from build123d import *

# Parameters (mm, degrees)
SKETCH1_W           = 41.2
SKETCH1_H           = 42
BOSS_EXTRUDE1_DEPTH = 5
CUT_EXTRUDE1_DEPTH  = 3
CUT_EXTRUDE2_DEPTH  = 2
SKETCH8_W           = 7.25
SKETCH8_H           = 6
BOSS_EXTRUDE4_DEPTH = 8
SKETCH9_W           = 7.25
SKETCH9_H           = 6
BOSS_EXTRUDE5_DEPTH = 8
SKETCH12_R          = 2
CUT_EXTRUDE4_DEPTH  = 6
BOSS_EXTRUDE6_DEPTH = 7.25
FILLET1_R           = 2
FILLET2_R           = 2


with BuildPart() as part:
    # Sketch1 → Boss-Extrude1 (new body)
    with BuildSketch(Plane.XY):
        with Locations((20.6, -21)):
            Rectangle(SKETCH1_W, SKETCH1_H)
    extrude(amount=BOSS_EXTRUDE1_DEPTH)

    # Sketch2 → Cut-Extrude1 (cut)
    with BuildSketch(Plane.XY.offset(5)):
        with BuildLine():
            Line((4, -2), (37.2, -2))
            ThreePointArc((37.2, -2), (38.614213562, -2.585786438), (39.2, -4))
            Line((39.2, -4), (39.2, -38))
            ThreePointArc((39.2, -38), (38.614213562, -39.414213562), (37.2, -40))
            Line((37.2, -40), (4, -40))
            ThreePointArc((4, -40), (2.585786438, -39.414213562), (2, -38))
            Line((2, -38), (2, -4))
            ThreePointArc((2, -4), (2.585786438, -2.585786438), (4, -2))
        make_face()
    extrude(amount=-CUT_EXTRUDE1_DEPTH, mode=Mode.SUBTRACT)

    # Sketch3 → Cut-Extrude2 (cut)
    with BuildSketch(Plane.XY.offset(2)):
        with BuildLine():
            Line((9.25, -7.25), (31.95, -7.25))
            ThreePointArc((31.95, -7.25), (33.364213562, -7.835786438), (33.95, -9.25))
            Line((33.95, -9.25), (33.95, -14.15))
            ThreePointArc((33.95, -14.15), (33.364213562, -15.564213562), (31.95, -16.15))
            Line((31.95, -16.15), (9.25, -16.15))
            ThreePointArc((9.25, -16.15), (7.835786438, -15.564213562), (7.25, -14.15))
            Line((7.25, -14.15), (7.25, -9.25))
            ThreePointArc((7.25, -9.25), (7.835786438, -7.835786438), (9.25, -7.25))
        make_face()
        with BuildLine():
            Line((9.25, -25.85), (31.95, -25.85))
            ThreePointArc((31.95, -25.85), (33.364213562, -26.435786438), (33.95, -27.85))
            Line((33.95, -27.85), (33.95, -32.75))
            ThreePointArc((33.95, -32.75), (33.364213562, -34.164213562), (31.95, -34.75))
            Line((31.95, -34.75), (9.25, -34.75))
            ThreePointArc((9.25, -34.75), (7.835786438, -34.164213562), (7.25, -32.75))
            Line((7.25, -32.75), (7.25, -27.85))
            ThreePointArc((7.25, -27.85), (7.835786438, -26.435786438), (9.25, -25.85))
        make_face()
    extrude(amount=-CUT_EXTRUDE2_DEPTH, mode=Mode.SUBTRACT)

    # Sketch8 → Boss-Extrude4 (add)
    with BuildSketch(Plane(origin=(0, 0, 0), x_dir=(-1, 0, 0), z_dir=(0, 0, -1))):
        with Locations((-37.575, -31)):
            Rectangle(SKETCH8_W, SKETCH8_H)
    extrude(amount=BOSS_EXTRUDE4_DEPTH)

    # Sketch9 → Boss-Extrude5 (add)
    with BuildSketch(Plane(origin=(0, 0, 0), x_dir=(-1, 0, 0), z_dir=(0, 0, -1))):
        with Locations((-3.625, -31)):
            Rectangle(SKETCH9_W, SKETCH9_H)
    extrude(amount=BOSS_EXTRUDE5_DEPTH)

    # Sketch12 → Cut-Extrude4 (cut)
    with BuildSketch(Plane(origin=(0, -28, 0), x_dir=(1, 0, 0), z_dir=(0, 1, 0))):
        with Locations(Location((37.575, 4, 0), (0, 0, 270))):
            Circle(SKETCH12_R)
    cut_extrude4 = extrude(amount=-CUT_EXTRUDE4_DEPTH, mode=Mode.SUBTRACT)

    # Sketch13 → Boss-Extrude6 (add)
    with BuildSketch(Plane(origin=(41.2, 0, 0), x_dir=(0, 0, -1), z_dir=(1, 0, 0))):
        Polygon((8, -28), (0, 0), (0, -28), align=None)
    boss_extrude6 = extrude(amount=-BOSS_EXTRUDE6_DEPTH)

    # Mirror2: Cut-Extrude4, Boss-Extrude6 across plane
    add(cut_extrude4.mirror(Plane(origin=(20.6, 0, 0), x_dir=(0, 0, 1), z_dir=(1, 0, 0))), mode=Mode.SUBTRACT)
    add(boss_extrude6.mirror(Plane(origin=(20.6, 0, 0), x_dir=(0, 0, 1), z_dir=(1, 0, 0))))

    # Fillet1
    fillet1_edges = [part.edges().sort_by_distance(p)[0] for p in [
        (0, 0, 2.5),
        (41.2, 0, 2.5),
        (41.2, -42, 2.5),
        (0, -42, 2.5),
    ]]
    fillet(fillet1_edges, radius=FILLET1_R)

    # Fillet2
    fillet2_edges = [part.edges().sort_by_distance(p)[0] for p in [
        (0, -31, -8),
        (7.25, -31, -8),
        (41.2, -31, -8),
        (33.95, -31, -8),
    ]]
    fillet(fillet2_edges, radius=FILLET2_R)


solid = part.part
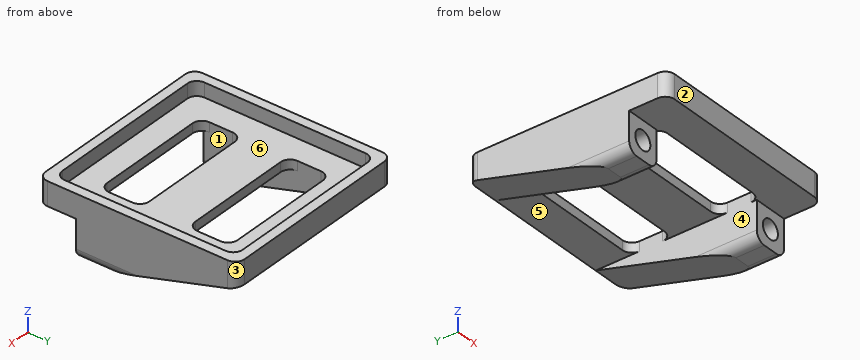
Source: CAD feature listing. Evaluate the final solid. Frame: model axes, mm. Face numbers are marked on the shaded views. A direction names the side the tool comes from. Give positions to 0.01 mm unless a question says otherwise; leave off trailing zeros. Order: outer loops, then holes, each group sorted by start corner. A loop starts at its lowest first (then second) coordinate and runs counter-clockwise, first axis right, second up. Notation, with made-up numbers: (84.5, 40.5) -> (122.5, 40.5) arc R10 cw to (122.5, 45.5) -> close; hole circle Ø1 at (24, 23). An arc over 180 degrees is marked (long way). Use a Markdown table: item, result.
1) Mould query, pull axis Y, two halves, no side actions, for the marked faces 1, 2 and 3. Classes: +Y half, -Y half, draft (parallel to the pull), parting line (faces both ways), or undercut.
Answer list:
| item | result |
|---|---|
| face 1 | undercut |
| face 2 | -Y half |
| face 3 | +Y half |
2) Contact query for flat-ended pins moving along their axis: P1, Ø1, axis at x = 6, y = -8, coming from the -Z side; P2, Ø7, axis at x = 25, y = -20, coming from the -Z side; P3, Ø3.5, axis at x = 4.5, z = -5.5, coming from the -Y side. Output: stop coordinate, or through.
Answer list:
| item | result |
|---|---|
| P1 | z = -2.43 |
| P2 | z = 0 |
| P3 | y = -34 |
3) Section query B-B, the plane z = 3. Return the cut outline in (x, y), then the cut area to 3 significant figures.
Answer list:
| item | result |
|---|---|
| outline | (0, -40) arc R2 ccw to (2, -42) -> (39.2, -42) arc R2 ccw to (41.2, -40) -> (41.2, -2) arc R2 ccw to (39.2, 0) -> (2, 0) arc R2 ccw to (0, -2) -> close; hole (2, -38) arc R2 ccw to (4, -40) -> (37.2, -40) arc R2 ccw to (39.2, -38) -> (39.2, -4) arc R2 ccw to (37.2, -2) -> (4, -2) arc R2 ccw to (2, -4) -> close |
| area | 317 mm² |
4) Reachability of the marked faces 4, 5 and 6 from +Z, -Z, +X, -X, +Y, -Y: full face, straight path, thin tool, end or side. Return the list, or none.
Answer list:
| item | result |
|---|---|
| face 4 | -Z |
| face 5 | -Z, +Y, -Y |
| face 6 | +Z |
5) Section query A-A, the plane z = -4. Return the cut outline in (x, y) (3 decimals).
Answer list:
| item | result |
|---|---|
| outline | (0, -34) -> (1.625, -34) -> (1.625, -28) -> (5.625, -28) -> (5.625, -34) -> (7.25, -34) -> (7.25, -14) -> (0, -14) -> close; (33.95, -34) -> (35.575, -34) -> (35.575, -28) -> (39.575, -28) -> (39.575, -34) -> (41.2, -34) -> (41.2, -14) -> (33.95, -14) -> close |
6) Section query C-C, the plane x = 8. Return the cut outline in (y, z), then the cut area to 3 significant figures.
Answer list:
| item | result |
|---|---|
| outline | (-42, 0) -> (-34.31, 0) -> (-34.31, 2) -> (-40, 2) -> (-40, 5) -> (-42, 5) -> close; (-26.29, 0) -> (-15.71, 0) -> (-15.71, 2) -> (-26.29, 2) -> close; (-7.69, 0) -> (0, 0) -> (0, 5) -> (-2, 5) -> (-2, 2) -> (-7.69, 2) -> close |
| area | 63.9 mm² |
7) Ray query, line 1 along X through (y, z) = (-32.75, -4) (3 decimals); line 2 along X through (y, z) = (-20, -3); line 3 along Y through (x, z) = (27.5, 3). Return the intervals inside material, ascending. Write a range as [from, to].
Answer list:
| item | result |
|---|---|
| line 1 | [0, 1.625], [5.625, 7.25], [33.95, 35.575], [39.575, 41.2] |
| line 2 | [0, 7.25], [33.95, 41.2] |
| line 3 | [-42, -40], [-2, 0] |
8) Section query D-D, the plane y = -11. Return the cut outline in (x, z), then the cut area to 3 significant figures.
Answer list:
| item | result |
|---|---|
| outline | (0, -3.14) -> (7.25, -3.14) -> (7.25, 2) -> (2, 2) -> (2, 5) -> (0, 5) -> close; (33.95, -3.14) -> (41.2, -3.14) -> (41.2, 5) -> (39.2, 5) -> (39.2, 2) -> (33.95, 2) -> close |
| area | 86.6 mm² |
